Study the drawing (mm; zero at the part's minimum x, y, z) and answer. Give positions to 0.01 mm unless a question says otherwise; leave off trailing zeros. Order: outer loops, then holes, each group sorted by start corner. A loop starts at its lowest first (then second) coordinate and runs counter-clockwise, first axis right, second up. Notation, with made-up numbers: (84, 31) -> (105, 31) arc R18 cw to (105, 60) -> close; hole circle Ø2 at (-19.5, 59). An arc over 180 degrees is marked (long way). Answer as CSV lines item,"result". Start each with the question number.
1. A cutting plane is placed at A-A (x = 30). Give the vertices of the cut face in (y, z), then the cut area to 3 significant figures.
2. For a pull along Z with two mould halves and no side action, classify the marked faces 1, 2 and 3 as released by +Z, released by -Z, zero draft, split by the parting line, or undercut.
3. A cutting plane is placed at B-B (z = 30). Give the vertices of the cut face in (x, y).
4. Flat-ended cylindrical pins translate along their axes: pin 1 (10 mm diameter, centred on x = 24.5, y = 14, fed in from -Z); pin 2 (1 mm diameter, centred on x = 43, z = 36, fed in from -Y); pin 3 (1.5 mm diameter, centred on x = 25.5, y = 12.5, fed in from -Z) (1 decimal); pin 4 (3 mm diameter, centred on x = 41.5, y = 7.5, fed in from -Z) (1 decimal). Find the tip coordinate at first contact, or state that the pin passes through.
5. A cutting plane is placed at C-C (y = 10.75). Give the vertices of the cut face in (x, z) (1 decimal), then the cut area to 3 significant figures.
6. A cutting plane is placed at D-D (x = 55). Give the vertices of the cut face in (y, z) (1 decimal).
7. Find the intervals of material crossed by L1, parallel to Z at x = 30, y = 15.75; L2, parallel to Z at x = 25, y = 18.25 (1 decimal); L3, parallel to X at y = 8, z = 22 (1 decimal), in increasing order.
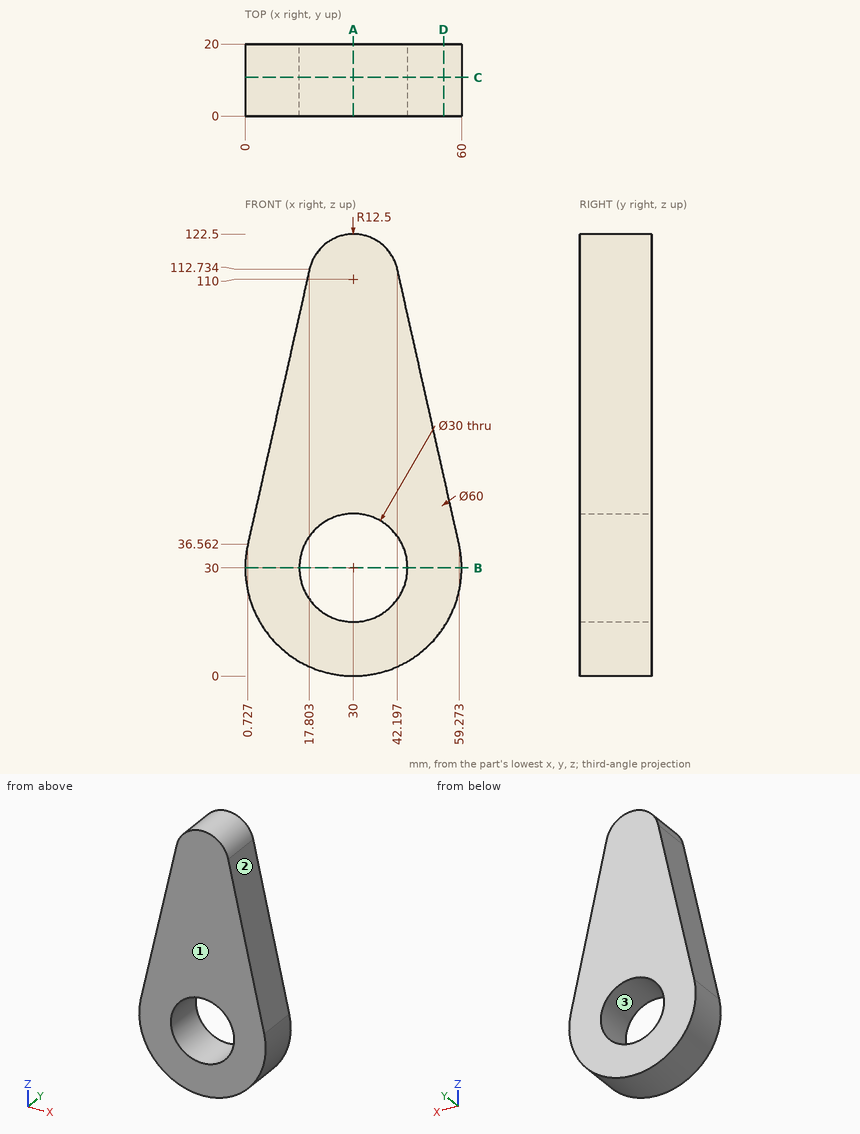
Answer sheet:
1,outline,"(0, 0) -> (20, 0) -> (20, 15) -> (0, 15) -> close; (0, 45) -> (20, 45) -> (20, 122.5) -> (0, 122.5) -> close"
1,area,"1,850 mm^2"
2,face 1,"zero draft"
2,face 2,"released by +Z"
2,face 3,"undercut"
3,outline,"(0, 0) -> (15, 0) -> (15, 20) -> (0, 20) -> close; (45, 0) -> (60, 0) -> (60, 20) -> (45, 20) -> close"
4,pin 1,"stops at z = 0"
4,pin 2,"passes through"
4,pin 3,"stops at z = 0.2"
4,pin 4,"stops at z = 1.7"
5,outline,"(0.7, 36.6) arc R30 ccw (long way) to (59.3, 36.6) -> (42.2, 112.7) arc R12.5 ccw to (17.8, 112.7) -> close; hole circle Ø30 at (30, 30)"
5,area,"4,430 mm^2"
6,outline,"(0, 13.4) -> (20, 13.4) -> (20, 55.6) -> (0, 55.6) -> close"
7,L1,"z = 0 to 15, 45 to 122.5"
7,L2,"z = 0.4 to 15.9, 44.1 to 121.5"
7,L3,"x = 1.1 to 17.3, 42.7 to 58.9"
